```python
from build123d import *

# Parameters (mm, degrees)
SKETCH3_W           = 277
SKETCH3_H           = 214
BOSS_EXTRUDE1_DEPTH = 14
FILLET1_R           = 30
CUT_EXTRUDE1_DEPTH  = 2
CUT_EXTRUDE2_DEPTH  = 2


with BuildPart() as part:
    # Sketch3 → Boss-Extrude1 (new body)
    with BuildSketch(Plane(origin=(0, 0, 0), x_dir=(1, 0, 0), z_dir=(0, 1, 0))):
        Rectangle(SKETCH3_W, SKETCH3_H)
    extrude(amount=BOSS_EXTRUDE1_DEPTH)

    # Fillet1
    fillet1_edges = [part.edges().sort_by_distance(p)[0] for p in [
        (138.5, 7, 107),
        (-138.5, 7, 107),
        (-138.5, 7, -107),
        (138.5, 7, -107),
    ]]
    fillet(fillet1_edges, radius=FILLET1_R)

    # Sketch4 → Cut-Extrude1 (cut)
    with BuildSketch(Plane(origin=(0, 14, 0), x_dir=(1, 0, 0), z_dir=(0, 1, 0))):
        with BuildLine():
            Line((-128.5, 77), (-128.5, -77))
            ThreePointArc((-128.5, -77), (-122.642135624, -91.142135624), (-108.5, -97))
            Line((-108.5, -97), (108.5, -97))
            ThreePointArc((108.5, -97), (122.642135624, -91.142135624), (128.5, -77))
            Line((128.5, -77), (128.5, 77))
            ThreePointArc((128.5, 77), (122.642135624, 91.142135624), (108.5, 97))
            Line((108.5, 97), (-108.5, 97))
            ThreePointArc((-108.5, 97), (-122.642135624, 91.142135624), (-128.5, 77))
        make_face()
    extrude(amount=-CUT_EXTRUDE1_DEPTH, mode=Mode.SUBTRACT)

    # Sketch5 → Cut-Extrude2 (cut)
    with BuildSketch(Plane.XZ):
        Polygon((-104.5, 96), (104.5, 96), (104.5, 77), (128.5, 77), (128.5, 0), (128.5, -77), (104.5, -77), (104.5, -96), (-104.5, -96), (-104.5, -77), (-128.5, -77), (-128.5, 77), (-104.5, 77), align=None)
    extrude(amount=-CUT_EXTRUDE2_DEPTH, mode=Mode.SUBTRACT)


solid = part.part
```
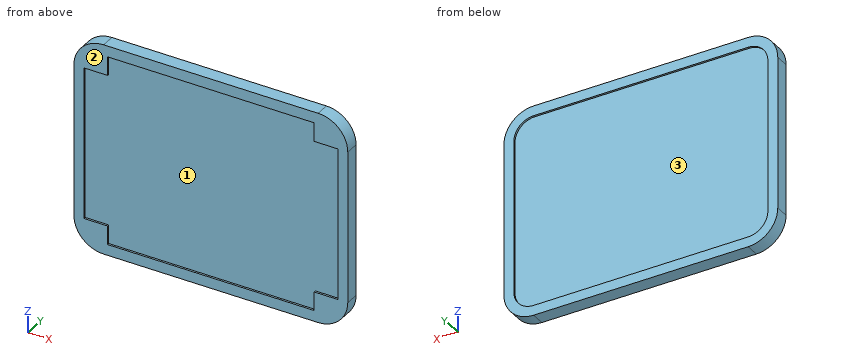
Can you work these out from the model? Positions are in its coordinate system, mm. Face numbers are marked on the shaded views. Give positions to 0.01 mm unless a question says otherwise; leave off trailing zeros. Loops run counter-clockwise (first coordinate to the right, second up) from the corner with the lowest first, then second, coordinate; pieces in that order, holes last. Notation, with made-up numbers: M 38,12.5 L 87,12.5 A15 cw 87,31.5 Z; hole C 10.25,-32.5 d8. An arc over 180 degrees is marked long. One line per item, written item: value.
(1) Will these pins go through, and if not, where does the flat tip stop? pin 1 (1 mm diameter, centred on x = 115, y = 1.5, fed in from -Z); pin 2 (0.6 mm diameter, centred on x = 114, y = 1, fed in from +Z); pin 3 (2 mm diameter, centred on y = 1, z = -88.5, fed in from -X).
Returned:
pin 1: z = -106.39
pin 2: z = 106.55
pin 3: x = -136.6
(2) I need wall thicknesses on line 1 (X direction, y = 13.25, z = -77); line 2 (Z direction, x = -27, y = 1.5); line 3 (Y direction, x = 83, z = -28). Which ranges of each line are inside material? Lowest first, please.
Returned:
line 1: -138.5 to -128.5, 128.5 to 138.5
line 2: -107 to -96, 96 to 107
line 3: 2 to 12
(3) Suppose I cut it at B-B on z = -16. List the corners of the cut face in (x, y) for me.
Returned:
outline: M -138.5,0 L -128.5,0 L -128.5,2 L 128.5,2 L 128.5,0 L 138.5,0 L 138.5,14 L 128.5,14 L 128.5,12 L -128.5,12 L -128.5,14 L -138.5,14 Z
(4) Suppose I cut it at A-A on x = 36. List the corners of the cut face in (y, z) for me.
Returned:
outline: M 0,-107 L 14,-107 L 14,-97 L 12,-97 L 12,97 L 14,97 L 14,107 L 0,107 L 0,96 L 2,96 L 2,-96 L 0,-96 Z
(5) We'd pull the mould along Z, two halves only. Please class the marked faces 1, 2 and 3: released by +Z, released by -Z, zero draft, split by the parting line, or undercut.
Returned:
face 1: undercut
face 2: zero draft
face 3: undercut
